For this review, take the finished solid that the model builds, in its own axes (mm). Face numbers are marked on the shaded views. A direction names the side the tool comes from. Give positions to 0.01 mm unless a question says otherwise; leave off trailing zeros. Loops run counter-clockwise (first coordinate to the right, second up) from the corner with the lowest first, then second, coordinate; pieces in that order, holes last.
```python
from build123d import *

# Parameters (mm, degrees)
BOSS_EXTRUDE3_DEPTH      = 4
BOSS_EXTRUDE3_DEPTH_BACK = 4
SKETCH11_R               = 0.85
CUT_EXTRUDE5_DEPTH       = 15.859761102


with BuildPart() as part:
    # Sketch6 → Boss-Extrude3 (new, two sides: drawn at the far end of the back side and taken through both)
    with BuildSketch(Plane.ZY.offset(-BOSS_EXTRUDE3_DEPTH_BACK)):
        Polygon((-4.75, 2), (-4.75, 0), (4.75, 0), (4.75, 2), (4, 11.5), (4, 13.5), (-4, 13.5), (-4, 11.5), align=None)
    extrude(amount=BOSS_EXTRUDE3_DEPTH + BOSS_EXTRUDE3_DEPTH_BACK)

    # Sketch11 → Cut-Extrude5 (cut, through all)
    with BuildSketch(Plane(origin=(0, 13.5, 0), x_dir=(1, 0, 0), z_dir=(0, 1, 0))):
        with Locations(Location((0, 0, 0), (0, 0, 270))):
            Circle(SKETCH11_R)
    extrude(amount=-CUT_EXTRUDE5_DEPTH, mode=Mode.SUBTRACT)


solid = part.part
```
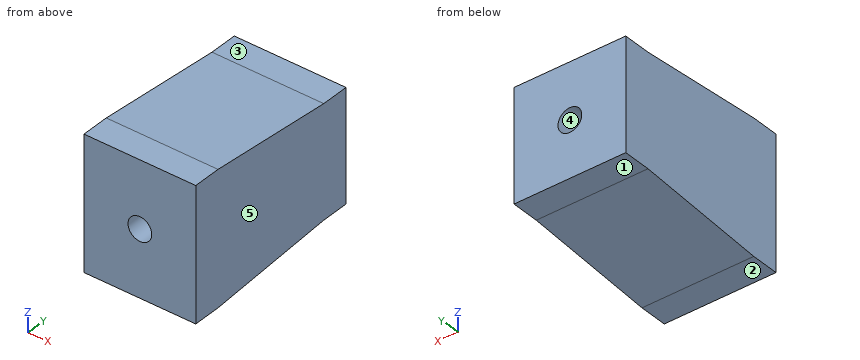
Item 1: Take a section at D-D on x = 2.5. Give the boundary of the cut face in (y, z), and give its area (3 significant figures).
Answer:
outline: (0, -4.75) - (2, -4.75) - (11.5, -4) - (13.5, -4) - (13.5, 4) - (11.5, 4) - (2, 4.75) - (0, 4.75) - close
area: 118 mm2
Item 2: The part is to be moulded in two halves that separate along X. For the marked faces 3, 4 and 5, say which applies: released by +X, released by -X, zero draft, split by the parting line, or undercut.
Answer:
face 3: zero draft
face 4: undercut
face 5: released by +X
Item 3: Take a section at A-A on z = 0. Give the boundary of the cut face in (x, y).
Answer:
outline: (-4, 0) - (-0.85, 0) - (-0.85, 13.5) - (-4, 13.5) - close; (0.85, 0) - (4, 0) - (4, 13.5) - (0.85, 13.5) - close
Item 4: Take a section at B-B on x = 0. Give the boundary of the cut face in (y, z), and give its area (3 significant figures).
Answer:
outline: (0, -4.75) - (2, -4.75) - (11.5, -4) - (13.5, -4) - (13.5, -0.85) - (0, -0.85) - close; (0, 0.85) - (13.5, 0.85) - (13.5, 4) - (11.5, 4) - (2, 4.75) - (0, 4.75) - close
area: 95.2 mm2
Item 5: Take a section at C-C on y = 1. Give the boundary of the cut face in (x, z), and give its area (3 significant figures).
Answer:
outline: (-4, -4.75) - (4, -4.75) - (4, 4.75) - (-4, 4.75) - close; hole circle Ø1.7 at (0, 0)
area: 73.7 mm2
Item 6: For L1, parallel to X at y = 3.5, z = 0; L2, parallel to Z at x = -0.5, y = 2.25; L3, parallel to X at y = 12, z = -0.75, list the stretches that pass through material, from the lowest coordinate up.
Answer:
L1: x = -4 to -0.85, 0.85 to 4
L2: z = -4.73 to -0.69, 0.69 to 4.73
L3: x = -4 to -0.4, 0.4 to 4
Item 7: Clearance check with flat-ended pins moving along their axes: pin 1 Ø1.4 at (x, z) = (0, 0) entering from +Y; pin 2 Ø4 at (x, y) = (1.5, 4.5) entering from -Z; pin 3 Ø0.6 at (x, y) = (0, 12.5) entering from +Z; pin 4 Ø2 at (x, y) = (-0.5, 13) entering from -Z. State where each tip first meets the part, or that it passes through.
Answer:
pin 1: passes through
pin 2: stops at z = -4.71
pin 3: stops at z = 4
pin 4: stops at z = -4
Item 8: Tool access review of the marked faces 1 and 2: name each direction out of +Z, -Z, +X, -X, +Y, -Y from which nothing blocks a thin tool from reaching the whole face with its end or side.
Answer:
face 1: -Z, +X, -X, +Y
face 2: -Z, +X, -X, +Y, -Y
